Input: part model. Units: mm. Frame: model coordinates. Face numbers are marked on the shaded views. A direction names the side the tool comes from. Give positions to 0.01 mm unless a question says otherwise; leave off trailing zeros. Loops run counter-clockwise (first coordinate to the right, second up) from the corner with the lowest first, then second, coordinate; pieces in that order, holes last. Notation, with made-up numbers: (84.5, 55) - (95.5, 55) arc R19 cw to (95.5, 78) - close; hole circle Ø6 at (49.5, 68). An arc over 180 degrees is marked (long way). One line per item, written item: value.
Autodesk Inventor part; units mm, degrees
ref_plane "YZ Plane" through (0, 0, 0) normal (1, 0, 0) x (0, 1, 0)
ref_plane "XZ Plane" through (0, 0, 0) normal (0, 1, 0) x (-1, 0, 0)
ref_plane "XY Plane" through (0, 0, 0) normal (0, 0, 1) x (1, 0, 0)
sketch "スケッチ1" plane through (0, 0, 0) normal (0, 0, 1) x (1, 0, 0)
  line L0 (0, 0) -> (0, 17.65)
  line L1 (0, 17.65) -> (28, 17.65)
  line L2 (28, 17.65) -> (28, 30.15)
  line L3 (28, 30.15) -> (58, 30.15)
  line L4 (58, 30.15) -> (58, 0)
  line L5 (58, 0) -> (60, 0)
  line L6 (60, 0) -> (60, 32.15)
  line L7 (60, 32.15) -> (28, 32.15)
  line L8 (28, 32.15) -> (26, 32.15)
  line L9 (26, 32.15) -> (26, 19.65)
  line L10 (26, 19.65) -> (-2, 19.65)
  line L11 (-2, 19.65) -> (-2, 0)
  line L12 (-2, 0) -> (0, 0)
  dimension "d0" = 17.65
  dimension "d1" = 28
  dimension "d2" = 12.5
  dimension "d3" = 30
  dimension "d4" = 2
  dimension "d5" = 32.15
  dimension "d6" = 32
  dimension "d7" = 2
  dimension "d8" = 12.5
  dimension "d9" = 28
extrude "押し出し1" add sketch "スケッチ1" along normal blind 14
sketch "スケッチ2" plane through (60, 0, 0) normal (1, 0, 0) x (0, 0, -1)
  line L0 (0, 0) -> (-14, 0)
  line L1 (-14, 0) -> (0, 0)
  line L2 (0, 0) -> (0, 2)
  line L3 (0, 2) -> (-14, 2)
  line L4 (-14, 2) -> (-14, 0)
  dimension "d12" = 14
  dimension "d13" = 2
extrude "押し出し2" add sketch "スケッチ2" along normal blind 7
sketch "スケッチ3" plane through (-2, 0, 0) normal (-1, 0, 0) x (0, 0, 1)
  line L0 (14, 2) -> (0, 2)
  line L1 (0, 0) -> (14, 0)
  line L2 (14, 0) -> (14, 2)
  line L3 (14, 2) -> (0, 2)
  line L4 (0, 2) -> (0, 0)
  dimension "d16" = 14
extrude "押し出し3" add sketch "スケッチ3" along normal blind 7
sketch "スケッチ4" plane through (0, 0, 14) normal (0, 0, 1) x (1, 0, 0)
  line L0 (60, 32.15) -> (60, 24.15)
  line L1 (60, 24.15) -> (61.6, 24.15)
  arc A0 (61.6, 20.4) -> (61.6, 27.9) centre (61.6, 24.15) ccw
  line L2 (61.6, 24.15) -> (61.6, 20.4) construction
  line L3 (61.6, 24.15) -> (61.6, 27.9) construction
  line L4 (61.6, 27.9) -> (60, 27.9)
  line L5 (61.6, 20.4) -> (60, 20.4)
  line L6 (60, 2) -> (60, 32.15)
  line L7 (60, 27.9) -> (60, 20.4)
  point P0 (0, 0)
  dimension "d47" = 8
  dimension "d48" = 1.6
  dimension "d49" = 3.75
  dimension "d50" = 180
extrude "押し出し4" add sketch "スケッチ4" against normal blind 14
hole "穴3" at (61.6, 24.15, 14) direction (0, 0, -1) diameter 3.75 end through all
sketch "スケッチ7" plane through (0, 0, 14) normal (0, 0, 1) x (1, 0, 0)
  line L0 (60, 32.15) -> (26, 32.15)
  line L1 (26, 32.15) -> (26, 24.15)
  line L2 (26, 24.15) -> (24.4, 24.15)
  arc A0 (24.4, 27.9) -> (24.4, 20.4) centre (24.4, 24.15) ccw
  line L3 (24.4, 27.9) -> (26, 27.9)
  line L4 (24.4, 20.4) -> (26, 20.4)
  line L5 (26, 20.4) -> (26, 27.9)
  line L6 (26, 32.15) -> (26, 19.65)
  circle A1 centre (24.4, 24.15) radius 1.875
  point P0 (0, 0)
  dimension "d60" = 8
  dimension "d61" = 1.6
  dimension "d62" = 3.75
  dimension "d63" = 3.75
extrude "押し出し6" add sketch "スケッチ7" against normal blind 14 contours L1 A1 L5 L4 A0 L3 | L1 L5 A1 picked at (23.6929, 24.15)
hole "穴4" at (24.4, 24.15, 14) direction (0, 0, -1) diameter 3.75 end through all
sketch "スケッチ10" plane through (0, 17.65, 0) normal (0, -1, 0) x (1, 0, 0)
  line L0 (28, 14) -> (58, 14)
  line L1 (0, 0) -> (28, 0)
  line L2 (28, 0) -> (28, 14)
  line L3 (28, 14) -> (0, 14)
  line L4 (0, 14) -> (0, 0)
extrude "押し出し7" cut sketch "スケッチ10" against normal blind 0.6
sketch "スケッチ11" plane through (0, 0, 0) normal (0, -1, 0) x (1, 0, 0)
  line L0 (0, 14) -> (-9, 14)
  line L1 (60, 0) -> (67, 0)
  line L2 (-9, 14) -> (67, 14)
  line L3 (67, 14) -> (67, 0)
  line L4 (67, 0) -> (-9, 0)
  line L5 (-9, 0) -> (-9, 14)
  point P0 (0, 0)
extrude "押し出し8" cut sketch "スケッチ11" against normal blind 0.6
sketch "スケッチ12" plane through (0, 0, 14) normal (0, 0, 1) x (1, 0, 0)
  line L0 (-2, 19.65) -> (-2, 2)
  line L1 (-2, 19.65) -> (4, 19.65)
  line L2 (26, 19.65) -> (-2, 19.65)
  line L3 (4, 19.65) -> (4, 18.25)
  line L4 (0, 18.25) -> (28, 18.25)
  line L5 (4, 18.25) -> (0.2844, 14.5344)
  line L6 (4, 18.25) -> (9.2547, 18.25) construction
  line L7 (0.2844, 14.5344) -> (0, 14.25)
  line L8 (0, 0.6) -> (0, 18.25)
  line L9 (0, 14.25) -> (-2, 14.25)
  line L10 (-2, 14.25) -> (-2, 19.65)
  point P0 (0, 0)
  dimension "d79" = 6
  dimension "d80" = 135
extrude "押し出し9" add sketch "スケッチ12" along normal blind 2
sketch "スケッチ15" plane through (0, 0, 0) normal (0, 0, -1) x (-1, 0, 0)
  line L0 (0, 0.6) -> (0, 18.25)
  line L1 (0, 18.25) -> (-14, 18.25)
  line L2 (-14, 18.25) -> (-14, 0.6)
  line L3 (-14, 0.6) -> (0, 0.6)
  line L4 (0, 0.6) -> (0, 18.25)
  point P0 (0, 0)
  dimension "d88" = 14
extrude "押し出し11" add sketch "スケッチ15" against normal blind 1.4
sketch "スケッチ17" plane through (67, 0, 0) normal (1, 0, 0) x (0, 0, -1)
  line L0 (0, 0.6) -> (-14, 0.6)
  line L1 (0, 0.6) -> (-14, 0.6)
  line L2 (-14, 0.6) -> (-14, 9.5309)
  line L3 (-14, 9.5309) -> (0, 9.5309)
  line L4 (0, 9.5309) -> (0, 0.6)
  point P0 (0, 0)
extrude "押し出し13" cut sketch "スケッチ17" against normal blind 3
sketch "スケッチ18" plane through (-9, 0, 0) normal (-1, 0, 0) x (0, 0, 1)
  line L0 (0, 0.6) -> (14, 0.6)
  line L1 (0, 0.6) -> (14, 0.6)
  line L2 (14, 0.6) -> (14, 6.5)
  line L3 (14, 6.5) -> (0, 6.5)
  line L4 (0, 6.5) -> (0, 0.6)
  point P0 (0, 0)
extrude "押し出し14" cut sketch "スケッチ18" against normal blind 3
hole "穴5" at (-4, 2, 7) direction (0, -1, 0) diameter 2.4 end through all
hole "穴6" at (62, 2, 7) direction (0, -1, 0) diameter 2.4 end through all
mirror "ミラー1" about plane through (31.8158, 20.0509, 0) normal (0, 0, -1) of "押し出し3", "押し出し1", "押し出し4", "穴3", "押し出し2", "穴6", "穴4", "押し出し6", "押し出し7", "押し出し9", "押し出し11", "押し出し14", "押し出し13", "穴5", "押し出し8"
sketch "スケッチ19" plane through (0, 0, 14) normal (0, 0, 1) x (1, 0, 0)
  line L0 (94.8832, 81.412) -> (-62.365, 81.412)
  line L1 (-62.365, 81.412) -> (-62.365, -71.7744)
  line L2 (-62.365, -71.7744) -> (94.8832, -71.7744)
  line L3 (94.8832, -71.7744) -> (94.8832, 81.412)
  point P0 (0, 0)
extrude "押し出し15" cut sketch "スケッチ19" against normal blind 14
sketch "スケッチ20" plane through (-2, 19.65, 14) normal (0, 1, 0) x (1, 0, 0)
  line L0 (17.6833, -4.2941) -> (-12.6138, -4.2941)
  line L1 (-12.6138, -4.2941) -> (-12.6138, 1.0873)
  line L2 (-12.6138, 1.0873) -> (17.6833, 1.0873)
  line L3 (17.6833, 1.0873) -> (17.6833, -4.2941)
  point P0 (2, 14)
extrude "押し出し16" cut sketch "スケッチ20" against normal blind 14
properties part number "センサ冶具2個積み右"
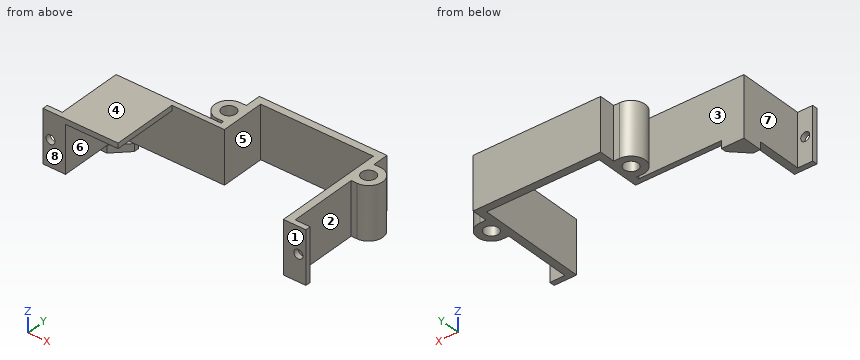
Item 1: Section D-D, the plane x = 30. Output: boundary loops of the cut face in (y, z), and give its area (3 significant figures).
Verdict:
outline: (30.15, -14) - (32.15, -14) - (32.15, 0) - (30.15, 0) - close
area: 28.0 mm^2
Item 2: Section A-A, the plane z = -7. Count the separate pieces of the cut face and the enclosed holes in it, and give its area (3 significant figures).
Verdict:
separate pieces: 3
enclosed holes: 2
area: 276 mm^2
Item 3: Pin query (flat end, axial travel): P1, Ø9.5, axis at y = 27, z = -9.5, coming from the +X side; P2, Ø4, axis at y = 11.5, z = -9.5, coming from the +X side; P3, Ø1.9, axis at x = 62, z = -7, coming from the -Y side; P4, Ø1, axis at y = 4.5, z = -4.5, coming from the -X side. Return the tip coordinate at first contact, or that it passes through.
Verdict:
P1: stops at x = 65.35
P2: stops at x = 60
P3: stops at y = 20.4
P4: stops at x = -2
Item 4: Section B-B, the plane x = -4. Output: boundary loops of the cut face in (y, z), and give its area (3 significant figures).
Verdict:
outline: (0.6, -14) - (2, -14) - (2, -8.2) - (0.6, -8.2) - close; (0.6, -5.8) - (2, -5.8) - (2, 0) - (0.6, 0) - close
area: 16.2 mm^2
Item 5: Access query for the marked faces 5, 6, 7 and 8. Directions: +Z, -Z, +X, -X, +Y, -Y. A direction counts if a zero-diameter tool reaches every point of the face in a straight line with its end or side. Return the directions, or none.
Verdict:
face 5: +Z, -Z, -Y
face 6: -Y
face 7: +Z, -Z, -X, +Y
face 8: +Z, -Z, +X, -X, -Y
Item 6: Section C-C, the plane y = 24.15. Output: boundary loops of the cut face in (x, z) (3 decimals).
Verdict:
outline: (20.65, -14) - (22.525, -14) - (22.525, 0) - (20.65, 0) - close; (26.275, -14) - (28, -14) - (28, 0) - (26.275, 0) - close; (58, -14) - (59.725, -14) - (59.725, 0) - (58, 0) - close; (63.475, -14) - (65.35, -14) - (65.35, 0) - (63.475, 0) - close
Item 7: Draft query along Y for the marked faces 1, 2, 3 and 4. Return one class per face: pulls with the +Y half, pulls with the -Y half, needs draft (parallel to the pull), parting line crosses it, or undercut.
Verdict:
face 1: pulls with the -Y half
face 2: undercut
face 3: undercut
face 4: needs draft
Item 8: Material intervals for L1, parallel to X at y = 24.15, z = -6.75 (3 decimals); L2, parallel to X at y = 1.15, z = -7; L3, parallel to X at y = 28, z = -5, sorted ascending.
Verdict:
L1: x = 20.65 to 22.525, 26.275 to 28, 58 to 59.725, 63.475 to 65.35
L2: x = -6 to -5.2, -2.8 to 0, 58 to 60.8, 63.2 to 64
L3: x = 26 to 28, 58 to 60
